from build123d import *

# Parameters (mm, degrees)
BOSS_EXTRUDE1_DEPTH = 19.05


with BuildPart() as part:
    # Sketch1 → Boss-Extrude1 (new body)
    with BuildSketch(Plane.XY):
        with BuildLine():
            Line((-228.088766336, -463.55), (-126.488766336, -463.55))
            Line((-126.488766336, -463.55), (-122.776078156, -463.55))
            ThreePointArc((-122.776078156, -463.55), (-118.207935902, -463.135837515), (-113.788766336, -461.906856405))
            ThreePointArc((-113.788766336, -461.906856405), (-102.527903247, -453.485299567), (-97.472732825, -440.363755866))
            Line((-97.472732825, -440.363755866), (-88.289138704, -335.394794733))
            ThreePointArc((-88.289138704, -335.394794733), (-84.217461675, -327.138250488), (-75.637466038, -323.801672666))
            Line((-75.637466038, -323.801672666), (-61.874871948, -323.801672666))
            Line((-61.874871948, -323.801672666), (61.874871948, -323.801672666))
            Line((61.874871948, -323.801672666), (75.637466038, -323.801672666))
            ThreePointArc((75.637466038, -323.801672666), (84.217461675, -327.138250488), (88.289138704, -335.394794733))
            Line((88.289138704, -335.394794733), (97.472732825, -440.363755866))
            ThreePointArc((97.472732825, -440.363755866), (102.527903247, -453.485299567), (113.788766336, -461.906856405))
            ThreePointArc((113.788766336, -461.906856405), (118.207935902, -463.135837515), (122.776078156, -463.55))
            Line((122.776078156, -463.55), (126.488766336, -463.55))
            Line((126.488766336, -463.55), (228.088766336, -463.55))
            Line((228.088766336, -463.55), (228.088766336, -273.05))
            Line((228.088766336, -273.05), (-228.088766336, -273.05))
            Line((-228.088766336, -273.05), (-228.088766336, -463.55))
        make_face()
    extrude(amount=BOSS_EXTRUDE1_DEPTH)


solid = part.part
CAD build for the part. Positions are in the model's coordinates, mm. A direction names the side the tool comes from. Give positions to 0.01 mm unless a question says otherwise; leave off trailing zeros. Write each loop counter-clockwise with the first axis right and the second up, starting at its lowest first coordinate (ties: lowest second). Pieces come first, ordered by that corner, then holes. Notation, with made-up numbers: M 5.25,-8 L 58.25,-8 A18 cw 58.25,20 Z; hole C 67.5,-15 d10. An arc over 180 degrees is marked long. Put each result on its own line as item: value. Start each with the question number.
(1) Flat gauge pins, fed straight in: pin 1 Ø5.5 at (x, z) = (-9.5, 10.5) entering from -Y; pin 2 Ø12 at (x, y) = (-157.5, -340.5) entering from -Z. Where does each tip first touch, or does it go through?
(2) Which spindle directions (+Z, -Z, +X, -X, +Y, -Y) get a long thin tool onto all of the face, cutting with end or side? Do faces 1 (the face through (-1, -323.802, 9)), 2 (the face through (3, -273.05, 9)). Say none if no direction does.
(3) Band-saw the part on B-B, the plane z = 6. Write the cut outline in (x, y).
(4) Band-saw the part on D-D, the plane x = 34.5. Write the cut outline in (y, z).
(5) Band-saw the part on A-A, the plane y = -429.5. Write the cut outline in (x, z), and give its area (3 significant figures).
(6) Band-saw the part on C-C, the plane y = -345. Write the cut outline in (x, z).
(7) Probe L1, parallel to Y at x = -48, z = 18; L2, parallel to X at y = -359, z = 15; L3, parallel to X at y = -407.5, z = 14.5. List the from-to ranges inside material, lowest first.
(8) Mould opens along X. For faces 3 (the face through (92.817, -387.144, 9.392)), 4 (the face through (-3, -303, 0)), 5 (the face through (-92.945, -388.614, 9.392)), 6 (the face through (228.089, -370, 9)) say: +X half, -X half, draft (parallel to the pull), parting line (faces both ways), or undercut.
Response values:
1. pin 1: stops at y = -323.8
1. pin 2: stops at z = 0
2. face 1: +Z, -Z, -Y
2. face 2: +Z, -Z, +X, -X, +Y
3. outline: M -228.09,-463.55 L -122.78,-463.55 A25.4 ccw -97.47,-440.36 L -88.29,-335.39 A12.7 cw -75.64,-323.8 L 75.64,-323.8 A12.7 cw 88.29,-335.39 L 97.47,-440.36 A25.4 ccw 122.78,-463.55 L 228.09,-463.55 L 228.09,-273.05 L -228.09,-273.05 Z
4. outline: M -323.8,0 L -273.05,0 L -273.05,19.05 L -323.8,19.05 Z
5. outline: M -228.09,0 L -96.52,0 L -96.52,19.05 L -228.09,19.05 Z; M 96.52,0 L 228.09,0 L 228.09,19.05 L 96.52,19.05 Z
5. area: 5,010 mm2
6. outline: M -228.09,0 L -89.13,0 L -89.13,19.05 L -228.09,19.05 Z; M 89.13,0 L 228.09,0 L 228.09,19.05 L 89.13,19.05 Z
7. L1: y = -323.8 to -273.05
7. L2: x = -228.09 to -90.35, 90.35 to 228.09
7. L3: x = -228.09 to -94.6, 94.6 to 228.09
8. face 3: undercut
8. face 4: draft
8. face 5: undercut
8. face 6: +X half
